from build123d import *

# Parameters (mm, degrees)
SKETCH1_R           = 27
SKETCH1_R_2         = 11.1125
SKETCH1_R_3         = 1.5
SKETCH1_R_4         = 15.1125
BOSS_EXTRUDE1_DEPTH = 3.175
CUT_EXTRUDE1_DEPTH  = 3.175
FILLET1_R           = 3


with BuildPart() as part:
    # Sketch1 → Boss-Extrude1 (new body)
    with BuildSketch(Plane.XY):
        Circle(SKETCH1_R)
        Circle(SKETCH1_R_2, mode=Mode.SUBTRACT)
        with Locations((15.909902577, 15.909902577)):
            Circle(SKETCH1_R_3, mode=Mode.SUBTRACT)
        with Locations((15.909902577, -15.909902577)):
            Circle(SKETCH1_R_3, mode=Mode.SUBTRACT)
        with Locations((-15.909902577, -15.909902577)):
            Circle(SKETCH1_R_3, mode=Mode.SUBTRACT)
        with Locations((-15.909902577, 15.909902577)):
            Circle(SKETCH1_R_3, mode=Mode.SUBTRACT)
        with BuildLine():
            ThreePointArc((15.1125, 121.52122), (-0.740058556, 106.426851196), (-15.040018721, 122.999561344))
            Line((-15.040018721, 122.999561344), (-26.87050491, 2.64120538))
            ThreePointArc((-26.87050491, 2.64120538), (0, 27), (26.87050491, 2.64120538))
            Line((26.87050491, 2.64120538), (15.040018721, 122.999561344))
            ThreePointArc((15.040018721, 122.999561344), (15.094368804, 122.261278556), (15.1125, 121.52122))
        make_face()
        with Locations((0, 121.52122)):
            Circle(SKETCH1_R_4)
        with Locations((0, 121.52122)):
            Circle(SKETCH1_R_2, mode=Mode.SUBTRACT)
    extrude(amount=BOSS_EXTRUDE1_DEPTH)

    # Sketch2 → Cut-Extrude1 (cut)
    with BuildSketch(Plane(origin=(0, 0, 0), x_dir=(-1, 0, 0), z_dir=(0, 0, -1))):
        with BuildLine():
            Line((21.005906623, 21.414723514), (-2.816362401, 106.673467339))
            ThreePointArc((-2.816362401, 106.673467339), (5.441374418, 107.422315763), (12.061107277, 112.415323695))
            Line((12.061107277, 112.415323695), (21.005906623, 21.414723514))
        make_face()
        Polygon((2.538490153, 65.851704894), (3.524956455, 67.930383746), (-8.266368844, 110.130964305), (-16.578304393, 25.568852363), align=None)
        with BuildLine():
            Line((16.957069467, 19.857503654), (5.165744168, 62.058084212))
            Line((5.165744168, 62.058084212), (-13.749853367, 22.199193423))
            ThreePointArc((-13.749853367, 22.199193423), (1.98555698, 26.036901116), (16.957069467, 19.857503654))
        make_face()
    extrude(amount=-CUT_EXTRUDE1_DEPTH, mode=Mode.SUBTRACT)

    # Fillet1
    fillet1_edges = [part.edges().sort_by_distance(p)[0] for p in [
        (2.816362401, 106.673467339, 1.5875),
        (-12.061107277, 112.415323695, 1.5875),
        (-21.005906623, 21.414723514, 1.5875),
        (8.266368844, 110.130964305, 1.5875),
        (-3.524956455, 67.930383746, 1.5875),
        (16.578304393, 25.568852363, 1.5875),
        (13.749853367, 22.199193423, 1.5875),
        (-5.165744168, 62.058084212, 1.5875),
        (-16.957069467, 19.857503654, 1.5875),
    ]]
    fillet(fillet1_edges, radius=FILLET1_R)


solid = part.part
The listing builds one solid part. Answer for the finished solid, in the listing's coordinates (mm). A direction names the side the tool comes from. Give positions to 0.01 mm unless a question says otherwise; leave off trailing zeros. Loops run counter-clockwise (first coordinate to the right, second up) from the corner with the lowest first, then second, coordinate; pieces in that order, holes last. Notation, with made-up numbers: M -24.75,84.5 L 12.25,84.5 A23 ccw 12.25,95.5 Z; hole C 64,59.5 d10. An arc over 180 degrees is marked long. Answer as CSV lines item,"result".
Item 1: The part is cut by section D-D (x = -22). Give the vertices of the cut face in (y, z) (3 decimals), and give its area (3 significant figures).
Values follow:
outline,"M -15.652,0 L 52.192,0 L 52.192,3.175 L -15.652,3.175 Z"
area,"215 mm^2"
Item 2: The part is cut by section B-B (z = 1.9). Give the number of separate pieces and of enclosed holes in the cut face, and give its area (3 significant figures).
Values follow:
separate pieces,"1"
enclosed holes,"9"
area,"4,170 mm^2"
Item 3: The part is cut by section C-C (y = 61). Give the vertices of the cut face in (x, z) (3 decimals), and give its area (3 significant figures).
Values follow:
outline,"M -21.134,0 L -17.115,0 L -17.115,3.175 L -21.134,3.175 Z; M -9.945,0 L -0.236,0 L -0.236,3.175 L -9.945,3.175 Z; M 13.096,0 L 21.134,0 L 21.134,3.175 L 13.096,3.175 Z"
area,"69.1 mm^2"
Item 4: Straight lines are drawn through the part: line 1 along Y through (x, z) = (9.5, 2.1); line 2 along X through (y, z) = (92, 0.35); line 3 along Y through (x, z) = (7, 2.1). For each, find the intervals that lie inside material, in ascending order. Write a range as [from, to].
Values follow:
line 1,"y = [-25.27, -5.77], [5.77, 25.75], [31.15, 40.62], [95.3, 115.76], [127.29, 133.27]"
line 2,"x = [-18.09, -14.07], [-1.28, 3.2], [10.05, 18.09]"
line 3,"y = [-26.08, -8.63], [8.63, 25.16], [36.42, 45.75], [96.9, 112.89], [130.15, 134.91]"
Item 5: Which of the six approach directions +Z, -Z, +X, -X, +Y, -Y give full straight-line access (tool end or side, diameter ignored) to faces 4 (the flat face through (-5.137, 78.208, 1.565)), 5 (the flat face through (12, 38, 3.175))?
Values follow:
face 4,"+Z, -Z"
face 5,"+Z, +X, -X, +Y, -Y"
Item 6: The part is cut by section A-A (y = 0). Give the vertices of the cut face in (x, z) (1 decimal).
Values follow:
outline,"M -27,0 L -11.1,0 L -11.1,3.2 L -27,3.2 Z; M 11.1,0 L 27,0 L 27,3.2 L 11.1,3.2 Z"
Item 7: The mould has two halves that part along X. Classify faces 1 (the cylindrical face through (0.31, 136.63, 1.57)), 2 (the flat face through (-20.872, 63.663, 1.565)), 3 (the flat face through (-15.11, 81.38, 1.57)): released by +X, released by -X, zero draft, split by the parting line, or undercut.
Values follow:
face 1,"split by the parting line"
face 2,"released by -X"
face 3,"undercut"
Item 8: Given pin 1 Ø1 at (x, z) = (-7, 3) entering from +Y; pin 2 Ø1 at (y, z) = (73, 1.5) entering from -X; pin 3 Ø2.5 at (x, y) = (-15.91, -15.91) entering from +Z, each flat-ended and moving along its own axis, determine where each tip first touches the part or whether it passes through.
Values follow:
pin 1,"stops at y = 135.16"
pin 2,"stops at x = -20"
pin 3,"passes through"
